from build123d import *

# Parameters (mm, degrees)
F0_W     = 131.865278
F0_H     = 127.425716
F1_DEPTH = 9.652
F2_R     = 79.271214
F3_DEPTH = 78.486
F4_R     = 69.127497
F5_DEPTH = 172.974
F7_DEPTH = 51.562
F9_DEPTH = 25.4


with BuildPart() as f1:
    # F0 (on Top) → F1 (new body)
    with BuildSketch(Plane.XY):
        Rectangle(F0_W, F0_H)
    extrude(amount=F1_DEPTH)

    # F2 (on face) → F3 (join)
    with BuildSketch(Plane(origin=(0, 0, 0), x_dir=(1, 0, 0), z_dir=(0, 0, -1))):
        with Locations((91.141589, 0)):
            Circle(F2_R)
    extrude(amount=-F3_DEPTH)

    # F4 (on face) → F5 (cut)
    with BuildSketch(Plane.XY.offset(78.486)):
        with Locations((91.141589, 0)):
            Circle(F4_R)
    extrude(amount=-F5_DEPTH, mode=Mode.SUBTRACT)

    # F6 (on face) → F7 (join)
    with BuildSketch(Plane.XY.offset(9.652)):
        with BuildLine():
            Line((-43.096259, 10.152509), (-43.096259, -11.246967))
            Line((-43.096259, -11.246967), (12.672289, -11.246967))
            ThreePointArc((12.672289, -11.246967), (11.872299, -0.552283), (12.523195, 10.152509))
            Line((12.523195, 10.152509), (-43.096259, 10.152509))
        make_face()
    extrude(amount=F7_DEPTH)

    # F8 (on face) → F9 (cut)
    with BuildSketch(Plane.XZ.offset(11.246967)):
        Polygon((-43.096259, 61.214), (-43.096259, 9.652), (12.672289, 61.214), align=None)
    extrude(amount=-F9_DEPTH, mode=Mode.SUBTRACT)


solid = f1.part
Input: part model. Units: mm. Frame: model coordinates. A direction names the side the tool comes from. Coordinates: 2 decimals unless noted, no trailing zeros. Loops run counter-clockwise (first coordinate to the right, second up) from the corner with the lowest first, then second, coordinate; pieces in that order, holes last.
Q1. Material intervals for line 1 (Y direction, x = 90, z = 10.5); line 2 (Y direction, x = 107, z = 60.5); line 3 (Z direction, x = -0.5, y = 56.5), sorted ascending.
Q2. Cut plane A-A (y = 0). Output: boundary loops of the cut face in (x, z).
Q3. Draft query along Y for faces 5 (the face through (-2, -1, 0)), 6 (the face through (-3, -11.247, 24)), 7 (the face through (82.14, 68.54, 39.79)). Return one class per face: +Y half, -Y half, draft (parallel to the pull), parting line (faces both ways), or undercut.
Q4. Set-up query: faces 1 (the face through (-9, 10.153, 29)), 2 (the face through (-12, -63.713, 5)), 3 (the face through (-24, 15, 9.652)), 4 (the face through (164.37, 30.36, 38.69)). Return all of +Z, -Z, +X, -X, +Y, -Y with unobstructed straight access to the full face (end or side cutting, diameter ignored); none if empty.
Q5. Cut plane C-C (z = 65). Output: boundary loops of the cut face in (x, y) (1 decimal), then the cut area to 3 significant figures.
Q6. Contact query for flat-ended pins moving along their axis: pin 1 (12 mm diameter, centred on y = 52, z = 10, fed in from +X); pin 2 (0.9 mm diameter, centred on x = 12.5, y = 3, fed in from -Z); pin 3 (3 mm diameter, centred on y = 55.5, z = 51, fed in from +X); pin 4 (5 mm diameter, centred on y = 62.5, z = 12, fed in from +X). Output: stop coordinate, or through.
Q7. Cut plane B-B (x = 24.5). Output: boundary loops of the cut face in (y, z).
Q8. Cut plane D-D (y = -59.5). Output: boundary loops of the cut face in (x, z), then the cut area to 3 significant figures.
Working result:
1. line 1: y = -79.26 to -69.12, 69.12 to 79.26
1. line 2: y = -77.67 to -67.28, 67.28 to 77.67
1. line 3: z = 0 to 9.65
2. outline: (-65.93, 0) - (22.01, 0) - (22.01, 78.49) - (11.87, 78.49) - (11.87, 61.21) - (12.67, 61.21) - (-43.1, 9.65) - (-65.93, 9.65) - close; (160.27, 0) - (170.41, 0) - (170.41, 78.49) - (160.27, 78.49) - close
3. face 5: draft
3. face 6: -Y half
3. face 7: undercut
4. face 1: +Z, -X, +Y
4. face 2: +Z, -Z, -X, -Y
4. face 3: +Z, -X
4. face 4: +Z
5. outline: circle Ø158.5 at (91.1, 0); hole circle Ø138.3 at (91.1, 0)
5. area: 4,730 mm2
6. pin 1: stops at x = 155.7
6. pin 2: stops at z = 0
6. pin 3: stops at x = 149.18
6. pin 4: stops at x = 142.95
7. outline: (-63.71, 0) - (-18.37, 0) - (-18.37, 78.49) - (-42.93, 78.49) - (-42.93, 9.65) - (-63.71, 9.65) - close; (18.37, 0) - (63.71, 0) - (63.71, 9.65) - (42.93, 9.65) - (42.93, 78.49) - (18.37, 78.49) - close
8. outline: (-65.93, 0) - (55.95, 0) - (55.95, 78.49) - (38.76, 78.49) - (38.76, 9.65) - (-65.93, 9.65) - close; (126.33, 0) - (143.52, 0) - (143.52, 78.49) - (126.33, 78.49) - close
8. area: 3,710 mm2
